For this review, take the finished solid that the model builds, in its own axes (mm). A direction names the side the tool comes from. Round coordinates to 2 decimals unless told otherwise and drop trailing zeros. Write each loop counter-clockwise with the first axis right and the second up, starting at its lowest first coordinate (ties: lowest second). Pieces come first, ordered by that corner, then holes. Notation, with made-up numbers: (69.25, -11) -> (101.25, -11) arc R22 ccw to (101.25, 18) -> close; hole circle Ø3 at (46, 72). An arc over 180 degrees is marked (long way). Answer in a Markdown table with one row per item.
from build123d import *

# Parameters (mm, degrees)
SKETCH1_W                    = 53.35524
SKETCH1_H                    = 1249.934
BASE_FLANGE1_DEPTH           = 1.89738
EDGE_FLANGE1_STRIP_W         = 11.65352
EDGE_FLANGE1_STRIP_H         = 1.89738
EDGE_FLANGE1_STRIP_CUT_DEPTH = 1249.934
EDGE_FLANGE1_DEPTH           = 1249.934
EDGE_FLANGE1_FLAT_DEPTH      = 1.89738
EDGE_FLANGE2_STRIP_W         = 11.65352
EDGE_FLANGE2_STRIP_H         = 1.89738
EDGE_FLANGE2_STRIP_CUT_DEPTH = 1249.934
EDGE_FLANGE2_DEPTH           = 1249.934
EDGE_FLANGE2_FLAT_DEPTH      = 1.89738
FILLET1_R                    = 2.54
SKETCH12_R                   = 2.4638
CUT_EXTRUDE1_DEPTH           = 629.39648529
SKETCH13_R                   = 2.4638
CUT_EXTRUDE2_DEPTH           = 629.39648529
SKETCH14_R                   = 2.4638
CUT_EXTRUDE3_DEPTH           = 629.39648529
F_1_2_0_5_DIAMETER_HOLE1_D   = 12.7


# Sheet-metal steps are written as plain solids
with BuildPart() as part:
    # Sketch1 → Base-Flange1 (new body)
    with BuildSketch(Plane.XY):
        Rectangle(SKETCH1_W, SKETCH1_H)
    extrude(amount=-BASE_FLANGE1_DEPTH)

    # Edge-Flange1 strip (across the edge) → Edge-Flange1 strip cut (cut)
    with BuildSketch(Plane(origin=(26.67762, 624.967, -1.89738), x_dir=(-1, 0, 0), z_dir=(0, -1, 0))):
        with Locations((-1.89738, -0.94869)):
            Rectangle(EDGE_FLANGE1_STRIP_W, EDGE_FLANGE1_STRIP_H)
    extrude(amount=EDGE_FLANGE1_STRIP_CUT_DEPTH, mode=Mode.SUBTRACT)

    # Edge-Flange1 bend section (across the edge) → Edge-Flange1 (add)
    with BuildSketch(Plane(origin=(26.67762, 624.967, -1.89738), x_dir=(-1, 0, 0), z_dir=(0, -1, 0))):
        with BuildLine():
            Line((0, 2.032), (1.89738, 2.032))
            ThreePointArc((1.89738, 2.032), (2.492539021, 0.595159021), (3.92938, 0))
            Line((3.92938, 0), (3.92938, -1.89738))
            ThreePointArc((3.92938, -1.89738), (1.150888756, -0.746491244), (0, 2.032))
        make_face()
    extrude(amount=EDGE_FLANGE1_DEPTH)

    # Edge-Flange1 profile (on flange) → Edge-Flange1 flat (add)
    with BuildSketch(Plane(origin=(26.67762, 0, -1.89738), x_dir=(0, 1, 0), z_dir=(-1, 0, 0))):
        Polygon((624.967, 2.032), (624.967, 2.87782), (619.090938633, 36.20262), (-624.967, 36.20262), (-624.967, 2.032), align=None)
    extrude(amount=EDGE_FLANGE1_FLAT_DEPTH)

    # Edge-Flange2 strip (across the edge) → Edge-Flange2 strip cut (cut)
    with BuildSketch(Plane(origin=(-26.67762, -624.967, -1.89738), x_dir=(1, 0, 0), z_dir=(0, 1, 0))):
        with Locations((-1.89738, -0.94869)):
            Rectangle(EDGE_FLANGE2_STRIP_W, EDGE_FLANGE2_STRIP_H)
    extrude(amount=EDGE_FLANGE2_STRIP_CUT_DEPTH, mode=Mode.SUBTRACT)

    # Edge-Flange2 bend section (across the edge) → Edge-Flange2 (add)
    with BuildSketch(Plane(origin=(-26.67762, -624.967, -1.89738), x_dir=(1, 0, 0), z_dir=(0, 1, 0))):
        with BuildLine():
            Line((0, 2.032), (1.89738, 2.032))
            ThreePointArc((1.89738, 2.032), (2.492539021, 0.595159021), (3.92938, 0))
            Line((3.92938, 0), (3.92938, -1.89738))
            ThreePointArc((3.92938, -1.89738), (1.150888756, -0.746491244), (0, 2.032))
        make_face()
    extrude(amount=EDGE_FLANGE2_DEPTH)

    # Edge-Flange2 profile (on flange) → Edge-Flange2 flat (add)
    with BuildSketch(Plane(origin=(-26.67762, 0, -1.89738), x_dir=(0, -1, 0), z_dir=(1, 0, 0))):
        Polygon((-624.967, 2.87782), (-624.967, 2.032), (624.967, 2.032), (624.967, 36.20262), (-619.090938633, 36.20262), align=None)
    extrude(amount=EDGE_FLANGE2_FLAT_DEPTH)

    # Fillet1
    fillet1_edges = [part.edges().sort_by_distance(p)[0] for p in [
        (25.72893, -624.967, -38.1),
        (25.72893, 619.090938633, -38.1),
        (-25.72893, -624.967, -38.1),
        (-25.72893, 619.090938633, -38.1),
    ]]
    fillet(fillet1_edges, radius=FILLET1_R)

    # Sketch12 → Cut-Extrude1 (cut, through all)
    with BuildSketch(Plane.ZY.offset(26.67762)):
        with Locations((-30.48, -617.347)):
            Circle(SKETCH12_R)
        with Locations((-30.48, -598.297)):
            Circle(SKETCH12_R)
        with Locations((-11.43, -598.297)):
            Circle(SKETCH12_R)
        with Locations((-11.43, -617.347)):
            Circle(SKETCH12_R)
    extrude(amount=-CUT_EXTRUDE1_DEPTH, mode=Mode.SUBTRACT)

    # Sketch13 → Cut-Extrude2 (cut, through all)
    with BuildSketch(Plane.ZY.offset(26.67762)):
        with Locations((-30.48, 612.696999444)):
            Circle(SKETCH13_R)
        with Locations((-11.43, 616.056028426)):
            Circle(SKETCH13_R)
        with Locations((-11.43, 596.71215147)):
            Circle(SKETCH13_R)
        with Locations((-30.48, 593.353122487)):
            Circle(SKETCH13_R)
    extrude(amount=-CUT_EXTRUDE2_DEPTH, mode=Mode.SUBTRACT)

    # Sketch14 → Cut-Extrude3 (cut, through all)
    with BuildSketch(Plane(origin=(26.67762, 0, 0), x_dir=(0, 0, -1), z_dir=(1, 0, 0))):
        with Locations((11.43, -313.817)):
            Circle(SKETCH14_R)
        with Locations((11.43, -332.867)):
            Circle(SKETCH14_R)
        with Locations((30.48, -332.867)):
            Circle(SKETCH14_R)
        with Locations((30.48, -313.817)):
            Circle(SKETCH14_R)
    extrude(amount=-CUT_EXTRUDE3_DEPTH, mode=Mode.SUBTRACT)

    # 1/2 (0.5) Diameter Hole1 (through all)
    with Locations(Plane.XY):
        with Locations((0, -504.317)):
            Hole(F_1_2_0_5_DIAMETER_HOLE1_D / 2)


solid = part.part
1) For line 1 (X direction, y = 236, z = -34); line 2 (Z direction, x = 8, y = 291.5); line 3 (Y direction, x = 0, z = -1.1), list the stretches that pass through material, from the lowest coordinate up. Write a range as [from, to].
Solved:
| item | result |
|---|---|
| line 1 | [-26.68, -24.78], [24.78, 26.68] |
| line 2 | [-1.9, 0] |
| line 3 | [-624.97, -510.67], [-497.97, 624.97] |
2) Consider section A-A on y = 228.5. State the section outline as (x, z) points, then the cut area to 3 significant figures.
Solved:
| item | result |
|---|---|
| outline | (-26.68, -38.1) -> (-24.78, -38.1) -> (-24.78, -3.93) arc R2.03 cw to (-22.75, -1.9) -> (22.75, -1.9) arc R2.03 cw to (24.78, -3.93) -> (24.78, -38.1) -> (26.68, -38.1) -> (26.68, -3.93) arc R3.93 ccw to (22.75, 0) -> (-22.75, 0) arc R3.93 ccw to (-26.68, -3.93) -> close |
| area | 234 mm² |
3) Clearance check with a flat-ended pin moving along its axis: pin 1 Ø2 at (x, y) = (-17.5, 480.5) entering from -Z. State where the tip first meets the part, or that it passes through.
Solved:
| item | result |
|---|---|
| pin 1 | z = -1.9 |
4) For faces 1 (the flat face through (26.678, -9, -21)), 2 (the flat face through (24.78, -9, -21)), list the 3-axis set-ups (+Z, -Z, +X, -X, +Y, -Y) from which the entire face can be reached by the end or side of a thin tool; tool diameter is ignored.
Solved:
| item | result |
|---|---|
| face 1 | +Z, -Z, +X, +Y, -Y |
| face 2 | -Z, +Y, -Y |
